Check sheet for the modelled part. Datum: model origin and axes. Units: mm. Face numbers are marked on the shaded views. Coordinates: 2 decimals unless noted, no trailing zeros. Write each loop counter-clockwise with the first axis right and the second up, starting at its lowest first coordinate (ties: lowest second). Pieces come first, ordered by that corner, then holes. Notation, with made-up numbers: M 41,1 L 50,1 A25 cw 50,30 Z; hole C -16,14.5 d6. An arc over 180 degrees is marked long. Answer as CSV lines item,"result". Start each with the question number.
1) Section check B-B (y = 4.25). Record the cut outline in (x, z), and give its area (3 significant figures).
2) Material ranges on L1, parallel to X at y = 3.75, z = 1.05; L2, parallel to Z at x = 15.75, y = 5.75; L3, parallel to Z at x = 14, y = 2.55, recorded low to high. Write a range as [from, to].
3) Draft check along X on the marked faces 1, 2, 3 and 4. Enter one of: +X half, -X half, draft (parallel to the pull), parting line (faces both ways), or undercut.
4) Section check A-A (z = 1.05). Record the cut outline in (x, y), and give its area (4 significant figures).
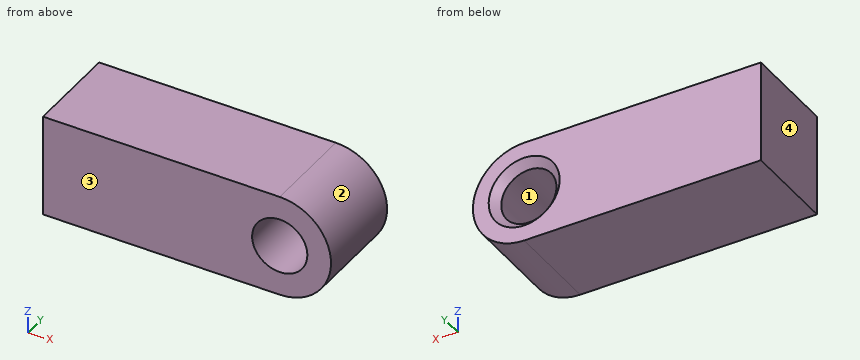
from build123d import *

# Parameters (mm, degrees)
SKETCH2_R           = 1.75
BOSS_EXTRUDE1_DEPTH = 6
CHAMFER1_SIZE       = 0.5
SKETCH3_W           = 11
SKETCH3_H           = 6
BOSS_EXTRUDE2_DEPTH = 2.2


with BuildPart() as part:
    # Sketch2 → Boss-Extrude1 (new body)
    with BuildSketch(Plane(origin=(0, 0, 0), x_dir=(1, 0, 0), z_dir=(0, 1, 0))):
        with BuildLine():
            Line((11, 2.2), (15, 2.2))
            ThreePointArc((15, 2.2), (18.25, -1.05), (15, -4.3))
            Line((15, -4.3), (0, -4.3))
            Line((0, -4.3), (0, 0))
            Line((0, 0), (11, 0))
            Line((11, 0), (11, 2.2))
        make_face()
        with Locations(Location((15, -1.05, 0), (0, 0, 270))):
            Circle(SKETCH2_R, mode=Mode.SUBTRACT)
    extrude(amount=BOSS_EXTRUDE1_DEPTH)

    # Chamfer1
    chamfer1_edges = [part.edges().sort_by_distance(p)[0] for p in [
        (15, 6, -0.7),
    ]]
    chamfer(chamfer1_edges, length=CHAMFER1_SIZE)

    # Sketch3 → Boss-Extrude2 (add)
    with BuildSketch(Plane(origin=(0, 0, 0), x_dir=(-1, 0, 0), z_dir=(0, 0, -1))):
        with Locations((-5.5, 3)):
            Rectangle(SKETCH3_W, SKETCH3_H)
    extrude(amount=BOSS_EXTRUDE2_DEPTH)


solid = part.part
Results found:
1,outline,"M 0,-2.2 L 15,-2.2 A3.25 ccw 15,4.3 L 0,4.3 Z; hole C 15,1.05 d3.5"
1,area,"104 mm2"
2,L1,"x = [0, 13.25], [16.75, 18.25]"
2,L2,"z = [-2.11, -0.8], [2.9, 4.21]"
2,L3,"z = [-2.2, -0.39], [2.49, 4.3]"
3,face 1,"undercut"
3,face 2,"+X half"
3,face 3,"draft"
3,face 4,"-X half"
4,outline,"M 0,0 L 13.25,0 L 13.25,5.5 L 12.75,6 L 0,6 Z; M 16.75,0 L 18.25,0 L 18.25,6 L 17.25,6 L 16.75,5.5 Z"
4,area,"88.25 mm2"
